Read the model definition and answer for the solid it produces. Units are mm, in the model's axes. Give positions to 0.01 mm unless a question says otherwise; leave off trailing zeros. Order: outer loops, then holes, each group sorted by start corner. A loop starts at its lowest first (then second) coordinate and runs counter-clockwise, first axis right, second up.
```python
from build123d import *

# Parameters (mm, degrees)
F1_DEPTH = 10
F1_TAPER = 2
F2_R     = 0.8
F3_DEPTH = 16
F4_R     = 0.4470893967
F5_DEPTH = 16.001
F7_W     = 2.1553949919
F7_H     = 1.9043667708
F8_DEPTH = 25


with BuildPart() as f1:
    # F0 (on Top) → F1 (new body)
    with BuildSketch(Plane.XY):
        Polygon((1, 4), (0, 4), (0, 0), (4, 0), (4, 1), (1, 1), align=None)
    extrude(amount=F1_DEPTH, taper=F1_TAPER)

    # F2 (on Top) → F3 (join)
    with BuildSketch(Plane.XY):
        with Locations((0.6, 0.6)):
            Circle(F2_R)
    extrude(amount=F3_DEPTH)

    # F4 (on face) → F5 (cut, through all)
    with BuildSketch(Plane.XY.offset(16)):
        with Locations((0.6, 0.6)):
            Circle(F4_R)
    extrude(amount=-F5_DEPTH, mode=Mode.SUBTRACT)

    # F7 (on face) → F8 (cut)
    with BuildSketch(Plane(origin=(2.0024329828, 1.9999985183, 8.50134e-05), x_dir=(0.7066765544, -0.7075367458, 3.0002e-05), z_dir=(-0.7075367451, -0.706676555, -3.00385e-05))):
        with Locations((-0.1619784161, 2.1438767435)):
            Rectangle(F7_W, F7_H)
    extrude(amount=F8_DEPTH, mode=Mode.SUBTRACT)


solid = f1.part
```
1) For a pull along Y with two mould halves and no side action, classify faces 1 (the face through (1.026, 0.734, 9.638)), 2 (the face through (1.026, 0.734, 0.604)), 3 (the face through (0.5, 1.5, 0)), 4 (the face through (-0.03, 0.11, 9.46)) as released by +Y, released by -Y, zero draft, split by the parting line, or undercut.
Final values:
face 1: undercut
face 2: undercut
face 3: zero draft
face 4: split by the parting line
2) Consider L1, parallel to Y at x = 0.6, z = 13.25; L2, parallel to Y at x = 0.9, z = 7.25; L3, parallel to X at y = 0.6, z = 8. Determine where each line is inside the solid, lowest interval first.
Final values:
L1: y = -0.2 to 0.15, 1.05 to 1.4
L2: y = -0.14 to 0.27, 0.93 to 1.34
L3: x = -0.2 to 0.15, 1.05 to 3.72
3) The part is cut by section A-A on z = 9.5. Determine the outline of the cut face in (x, y).
Final values:
outline: (0.33, 1.35) arc R0.8 ccw (long way) to (1.35, 0.33) - (3.67, 0.33) - (3.67, 0.67) - (1.4, 0.67) arc R0.8 ccw to (0.67, 1.4) - (0.67, 3.67) - (0.33, 3.67) - close; hole circle Ø0.89 at (0.6, 0.6)
4) Given pin 1 (1.5 mm diameter, centred on y = 3, z = 9.5, fed in from +X), flat-ended and moving along its own axis, determine where the tip first touches the part or whether it passes through.
Final values:
pin 1: stops at x = 0.69
5) The part is cut by section B-B on y = 1.6. Determine the outline of the cut face in (x, z), and give its area (3 significant figures).
Final values:
outline: (0, 0) - (1, 0) - (0.96, 1.19) - (0.04, 1.19) - close; (0.11, 3.1) - (0.89, 3.1) - (0.65, 10) - (0.35, 10) - close
area: 4.89 mm2
6) The part is cut by section C-C on x = 2.45. Determine the outline of the cut face in (y, z), and give its area (3 significant figures).
Final values:
outline: (0, 0) - (1, 0) - (0.65, 10) - (0.35, 10) - close
area: 6.51 mm2
7) The part is cut by section D-D on z = 12.5. Determine the outline of the cut face in (x, y).
Final values:
outline: circle Ø1.6 at (0.6, 0.6); hole circle Ø0.89 at (0.6, 0.6)
